Can you work these out from the model? Positions are in its coordinate system, mm. Face numbers are marked on the shaded views. A direction names the side the tool comes from. Coordinates: 2 decimals unless noted, no trailing zeros. Loops run counter-clockwise (first coordinate to the right, second up) from the corner with the lowest first, then second, coordinate; pieces in that order, holes last. Notation, with made-up numbers: M 24,86 L 82,86 A23 cw 82,124 Z; hole C 25,44 d8. An arc over 180 degrees is marked long. Answer as a JSON object with one key per item and string values. Group by question number.
Item 1: If I drill on line 1 (X direction, y = 4.75, z = 2); line 2 (Y direction, x = 29, z = 15.75); line 3 (X direction, y = -1.25, z = 21), over which ranges is the centre line in solid material (lowest first)?
Item 2: Suppose I cut it at A-A (y = 4.25). Write out the boundary of the cut face in (x, z).
Item 3: Which directions (+Z, -Z, +X, -X, +Y, -Y) give clear straight access to the entire face, cutting with the end or side of a thin tool? Please do the marked faces 4, 5 and 6.
Item 4: I'm going to push flat-ended pins straight in: pin 1 Ø1.5 at (y, z) = (4, 10.5) entering from -X; pin 2 Ø1.5 at (y, z) = (3, 15.5) entering from +X; pin 3 Ø12 at (x, z) = (0, 12.5) entering from -Y. Where does each tip first touch, or does it pass through?
Item 5: Suppose I cut it at B-B (z = 12.5). Write out the boundary of the cut face in (x, y), then the cut area to 3 significant figures.
Item 6: Suppose I cut it at D-D (z = 20). Write out the boundary of the cut face in (x, y), then the cut area to 3 significant figures.
Item 7: Suppose I cut it at C-C (x = 0). Write out the boundary of the cut face in (y, z).
Item 8: We'd pull the mould along X, two halves only. Please class the marked faces 1, 2 and 3: +X half, -X half, draft (parallel to the pull), parting line (faces both ways), or undercut.
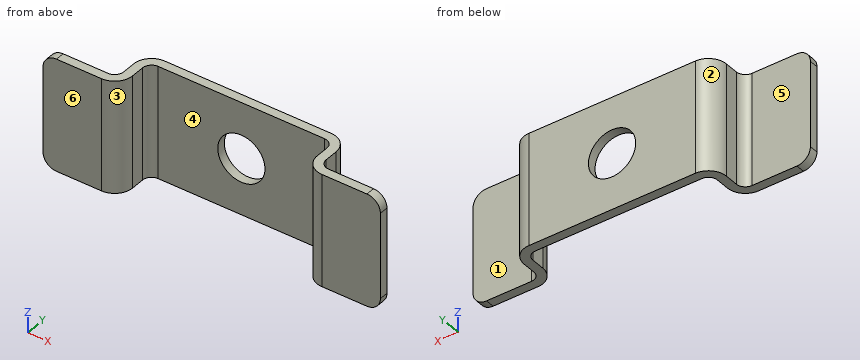
```python
from build123d import *

# Parameters (mm, degrees)
BASE_FLANGE1_DEPTH = 25
SKETCH7_R          = 5.25
CUT_EXTRUDE1_DEPTH = 10
FILLET1_R          = 3


# Sheet-metal steps are written as plain solids
with BuildPart() as part:
    # Sketch1 → Base-Flange1 (new body)
    with BuildSketch(Plane.XY):
        with BuildLine():
            Line((-37.5, 0), (-24.5, 0))
            ThreePointArc((-24.5, 0), (-23.085786438, 0.585786438), (-22.5, 2))
            Line((-22.5, 2), (-22.5, 5))
            ThreePointArc((-22.5, 5), (-21.328427125, 7.828427125), (-18.5, 9))
            Line((-18.5, 9), (18.5, 9))
            ThreePointArc((18.5, 9), (21.328427125, 7.828427125), (22.5, 5))
            Line((22.5, 5), (22.5, 2))
            ThreePointArc((22.5, 2), (23.085786438, 0.585786438), (24.5, 0))
            Line((24.5, 0), (37.5, 0))
            Line((37.5, 0), (37.5, -2))
            Line((37.5, -2), (24.5, -2))
            ThreePointArc((24.5, -2), (21.671572875, -0.828427125), (20.5, 2))
            Line((20.5, 2), (20.5, 5))
            ThreePointArc((20.5, 5), (19.914213562, 6.414213562), (18.5, 7))
            Line((18.5, 7), (-18.5, 7))
            ThreePointArc((-18.5, 7), (-19.914213562, 6.414213562), (-20.5, 5))
            Line((-20.5, 5), (-20.5, 2))
            ThreePointArc((-20.5, 2), (-21.671572875, -0.828427125), (-24.5, -2))
            Line((-24.5, -2), (-37.5, -2))
            Line((-37.5, -2), (-37.5, 0))
        make_face()
    extrude(amount=BASE_FLANGE1_DEPTH)

    # Sketch7 → Cut-Extrude1 (cut)
    with BuildSketch(Plane(origin=(0, 9, 0), x_dir=(1, 0, 0), z_dir=(0, 1, 0))):
        with Locations(Location((0, -12.5, 0), (0, 0, 270))):
            Circle(SKETCH7_R)
    extrude(amount=-CUT_EXTRUDE1_DEPTH, mode=Mode.SUBTRACT)

    # Fillet1
    fillet1_edges = [part.edges().sort_by_distance(p)[0] for p in [
        (-37.5, -1, 0),
        (37.5, -1, 0),
        (-37.5, -1, 25),
        (37.5, -1, 25),
    ]]
    fillet(fillet1_edges, radius=FILLET1_R)


solid = part.part
```
From the geometry:
{
 "1": {"line 1": "-22.5 to -20.5, 20.5 to 22.5", "line 2": "-2 to 0", "line 3": "-37.5 to -22.17, 22.17 to 37.5"},
 "2": {"outline": "M -22.5,0 L -20.5,0 L -20.5,25 L -22.5,25 Z; M 20.5,0 L 22.5,0 L 22.5,25 L 20.5,25 Z"},
 "3": {"face 4": "+Z, -Z, -Y", "face 5": "+Z, -Z, -X, +Y", "face 6": "+Z, -Z, +X, -X, -Y"},
 "4": {"pin 1": "x = -22.5", "pin 2": "x = 22.5", "pin 3": "y = 7"},
 "5": {"outline": "M -37.5,-2 L -24.5,-2 A4 ccw -20.5,2 L -20.5,5 A2 cw -18.5,7 L -5.25,7 L -5.25,9 L -18.5,9 A4 ccw -22.5,5 L -22.5,2 A2 cw -24.5,0 L -37.5,0 Z; M 5.25,7 L 18.5,7 A2 cw 20.5,5 L 20.5,2 A4 ccw 24.5,-2 L 37.5,-2 L 37.5,0 L 24.5,0 A2 cw 22.5,2 L 22.5,5 A4 ccw 18.5,9 L 5.25,9 Z", "area": "155 mm2"},
 "6": {"outline": "M -37.5,-2 L -24.5,-2 A4 ccw -20.5,2 L -20.5,5 A2 cw -18.5,7 L 18.5,7 A2 cw 20.5,5 L 20.5,2 A4 ccw 24.5,-2 L 37.5,-2 L 37.5,0 L 24.5,0 A2 cw 22.5,2 L 22.5,5 A4 ccw 18.5,9 L -18.5,9 A4 ccw -22.5,5 L -22.5,2 A2 cw -24.5,0 L -37.5,0 Z", "area": "176 mm2"},
 "7": {"outline": "M 7,0 L 9,0 L 9,7.25 L 7,7.25 Z; M 7,17.75 L 9,17.75 L 9,25 L 7,25 Z"},
 "8": {"face 1": "draft", "face 2": "-X half", "face 3": "undercut"}
}
